Geometry check sheet. Reference: drawing and pictorial views, mm from the part's lowest x, y, z. A direction names the side the tool comes from. Round coordinates to 2 decimals unless told otherwise and drop trailing zeros. Write each loop counter-clockwise with the first axis right and the second up, starting at its lowest first coordinate (ties: lowest second). Pieces come first, ordered by that corner, then holes. Notation, with made-up numbers: M 35.5,-11.75 L 63.5,-11.75 A29 cw 63.5,14.25 Z; hole C 29,-22.5 d6. An arc over 180 degrees is marked long. One line per item, written item: value. Start each with the question number.
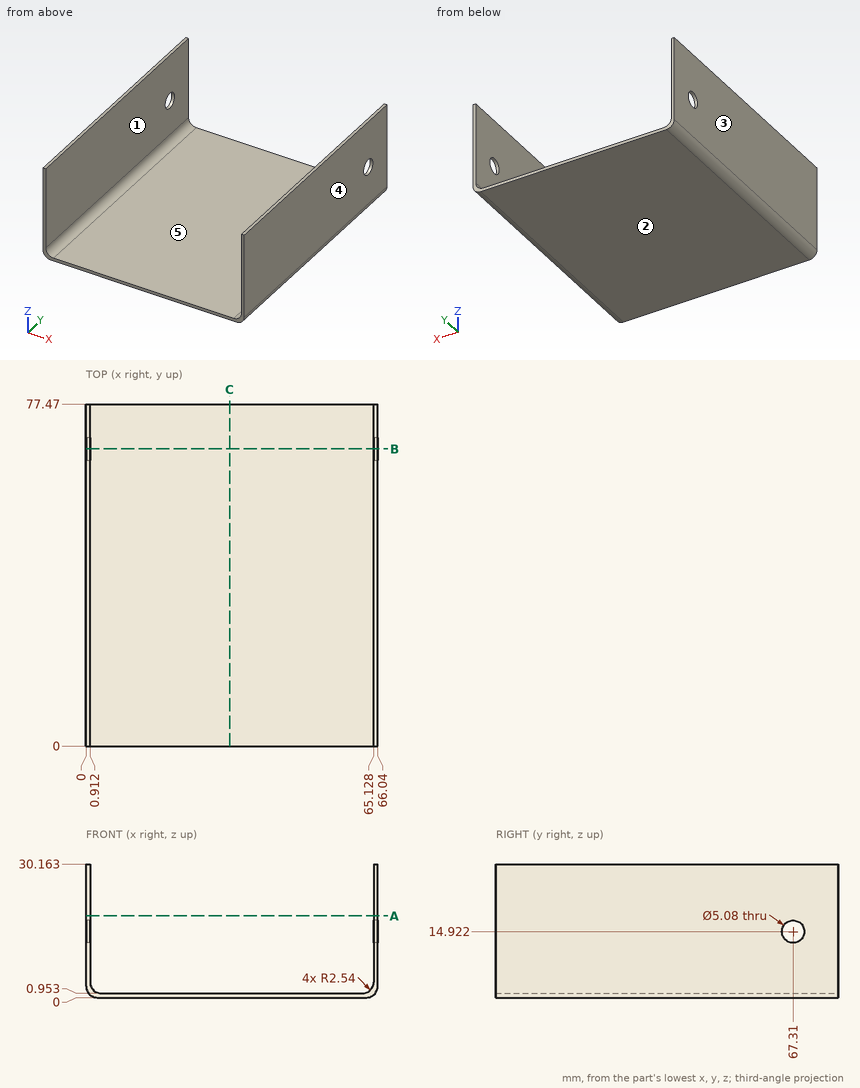
1) Mould release check, pull along X, two halves, no side actions. Record for the marked faces 1, 2 and 3: pulls with the +X half, pulls with the -X half, needs draft (parallel to the pull), parting line crosses it, or undercut.
2) Thickness scan on line 1 (X direction, y = 19, z = 23); line 2 (Z direction, x = 30, y = 40); line 3 (Z direction, x = 0.25, y = 67.31) (1 decimal). Record the ranges inside material, lowest first.
3) Gauge pin test, flat ends, axial feed: pin 1 Ø8 at (x, y) = (39, 36) entering from +Z; pin 2 Ø3 at (y, z) = (67.31, 14.92) entering from -X. Record the tip position at first contact, or that the pin passes through.
4) Access from +Z, -Z, +X, -X, +Y, -Y to the whole of each face (thin tool, end or side, straight path). Record for the marked faces 4 and 5.
5) Cross-section at B-B (y = 67.31). Record the boundary of the cut face in (x, z).
6) Cross-section at C-C (x = 32.5). Record the boundary of the cut face in (y, z).
7) Cross-section at A-A (z = 18.5). Record the boundary of the cut face in (x, y).
Results below:
1. face 1: undercut
1. face 2: needs draft
1. face 3: pulls with the -X half
2. line 1: x = 0 to 0.91, 65.13 to 66.04
2. line 2: z = 0 to 0.95
2. line 3: z = 1.4 to 12.4, 17.5 to 30.2
3. pin 1: stops at z = 0.95
3. pin 2: passes through
4. face 4: +Z, -Z, +X, +Y, -Y
4. face 5: +Z, +Y, -Y
5. outline: M 0,2.54 A2.54 ccw 2.54,0 L 63.5,0 A2.54 ccw 66.04,2.54 L 66.04,12.38 L 65.13,12.38 L 65.13,3.49 A2.54 cw 62.59,0.95 L 3.45,0.95 A2.54 cw 0.91,3.49 L 0.91,12.38 L 0,12.38 Z; M 0,17.46 L 0.91,17.46 L 0.91,30.16 L 0,30.16 Z; M 65.13,17.46 L 66.04,17.46 L 66.04,30.16 L 65.13,30.16 Z
6. outline: M 0,0 L 77.47,0 L 77.47,0.95 L 0,0.95 Z
7. outline: M 0,0 L 0.91,0 L 0.91,77.47 L 0,77.47 Z; M 65.13,0 L 66.04,0 L 66.04,77.47 L 65.13,77.47 Z
